Geometry: final body of the model. Coordinates: model frame, mm. Coordinates: 2 decimals unless noted, no trailing zeros. Write each loop counter-clockwise with the first axis right and the second up, starting at its lowest first coordinate (ties: lowest second). Pieces come first, ordered by that corner, then holes. Notation, with made-up numbers: (33.25, -3) -> (86.25, -3) arc R34 cw to (86.25, 30) -> close; hole circle Ø2 at (27, 41). An arc over 180 degrees is marked (long way). One line per item, written item: value.
Autodesk Inventor part; units mm, degrees
ref_plane "YZ Plane" through (0, 0, 0) normal (1, 0, 0) x (0, 1, 0)
ref_plane "XZ Plane" through (0, 0, 0) normal (0, 1, 0) x (-1, 0, 0)
ref_plane "XY Plane" through (0, 0, 0) normal (0, 0, 1) x (1, 0, 0)
sketch "Sketch1" plane through (0, 0, 0) normal (0, 1, 0) x (-1, 0, 0)
  line L0 (10.75, 21.75) -> (-10.75, 21.75)
  line L1 (-10.75, 21.75) -> (-10.75, -21.75)
  line L2 (-10.75, -21.75) -> (10.75, -21.75)
  line L3 (10.75, -21.75) -> (10.75, 21.75)
  line L4 (10.75, 21.75) -> (-10.75, -21.75) construction
  line L5 (-10.75, 21.75) -> (10.75, -21.75) construction
  line L6 (8, -15.25) -> (-8, -15.25) construction
  line L7 (-8, -15.25) -> (-8, 15.25) construction
  line L8 (-8, 15.25) -> (8, 15.25) construction
  line L9 (8, 15.25) -> (8, -15.25) construction
  line L10 (8, -15.25) -> (-8, 15.25) construction
  line L11 (-8, -15.25) -> (8, 15.25) construction
  circle A0 centre (8, 15.25) radius 1.65
  circle A1 centre (-8, -15.25) radius 1.65
  point P0 (0, 0)
  dimension "d0" = 21.5
  dimension "d1" = 43.5
  dimension "d2" = 16
  dimension "d3" = 30.5
  dimension "d4" = 3.3
  dimension "d5" = 3.3
extrude "Extrusion1" add sketch "Sketch1" along normal blind 0.5
(1) Line query: line 1 (Z direction, x = 8, y = 0.35); line 2 (X direction, y = 0.1, z = -14.5); line 3 (Z direction, x = -8, y = 0.3). Output: solid intervals per line, ascending. Write a range as [from, to].
Responses:
line 1: z = [-21.75, -16.9], [-13.6, 21.75]
line 2: x = [-10.75, 6.53], [9.47, 10.75]
line 3: z = [-21.75, 13.6], [16.9, 21.75]
(2) Pull-direction query (X, two-part tool) for faces 1 (the flat face through (0, 0, 0)), 2 (the cylindrical face through (-6.784, 0.246, 14.135)), 3 (the cylindrical face through (9.65, 0.25, -15.32)); classes: released by +X, released by -X, zero draft, split by the parting line, or undercut.
Responses:
face 1: zero draft
face 2: undercut
face 3: undercut
(3) Section B-B (z = -15.25). Return the cut outline in (x, y), then the cut area to 3 significant figures.
Responses:
outline: (-10.75, 0) -> (6.35, 0) -> (6.35, 0.5) -> (-10.75, 0.5) -> close; (9.65, 0) -> (10.75, 0) -> (10.75, 0.5) -> (9.65, 0.5) -> close
area: 9.10 mm2
(4) Section C-C (y = 0.3). Return the cut outline in (x, z), then the cut area to 3 significant figures.
Responses:
outline: (-10.75, -21.75) -> (10.75, -21.75) -> (10.75, 21.75) -> (-10.75, 21.75) -> close; hole circle Ø3.3 at (-8, 15.25); hole circle Ø3.3 at (8, -15.25)
area: 918 mm2
(5) Section A-A (x = -8). Return the cut outline in (y, z).
Responses:
outline: (0, -21.75) -> (0.5, -21.75) -> (0.5, 13.6) -> (0, 13.6) -> close; (0, 16.9) -> (0.5, 16.9) -> (0.5, 21.75) -> (0, 21.75) -> close
